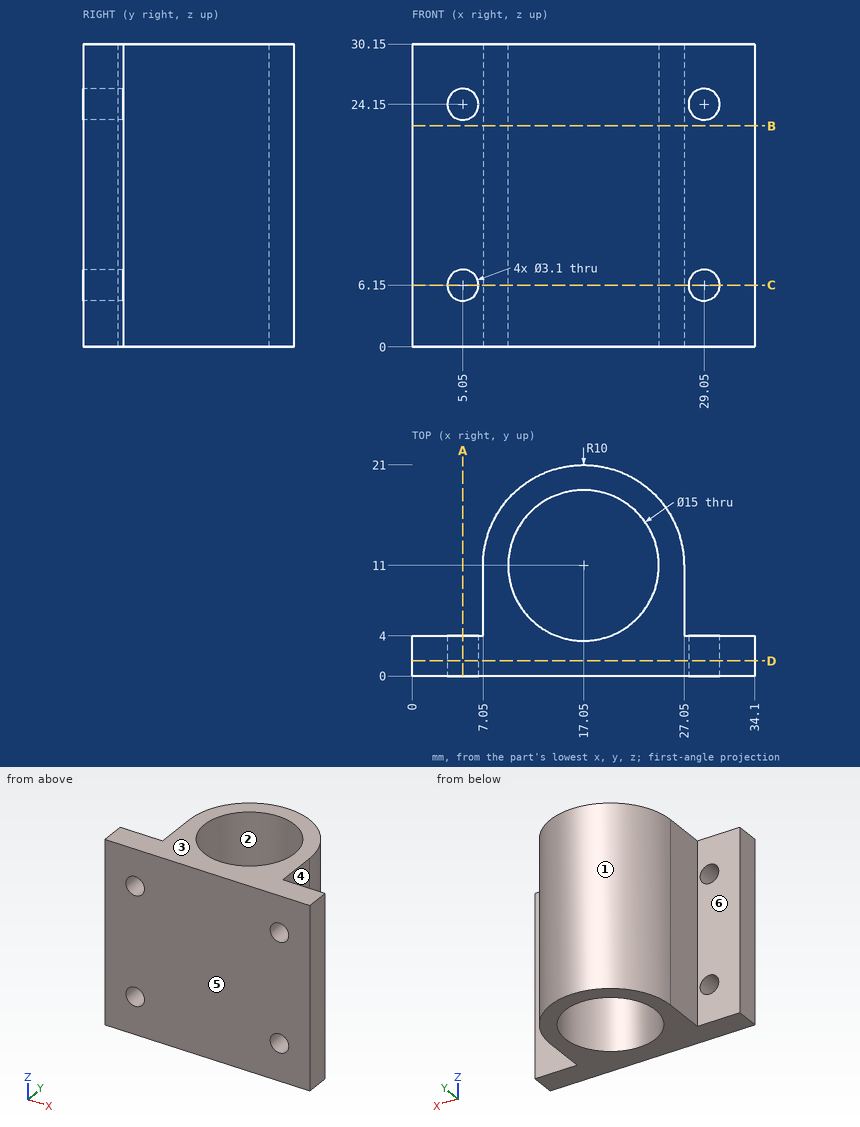
Job drawing, mm, ordinate dimensions from the low corner. One solid piece. A direction names the side the tool comes from. Coordinates: 2 decimals unless noted, no trailing zeros. Write each loop counter-clockwise with the first axis right and the second up, starting at its lowest first coordinate (ties: lowest second). Pieces come first, ordered by that corner, then holes.
Item 1: Slice it at A-A (x = 5.05). Write the cut outline in (y, z), and give its area (3 significant figures).
Item 2: Mould opens along X. For the marked faces 1, 2 and 3 say: released by +X, released by -X, zero draft, split by the parting line, or undercut.
Item 3: Slice it at D-D (y = 1.5). Write the cut outline in (x, z).
Item 4: Slice it at B-B (z = 22). Write the cut outline in (x, y).
Item 5: Probe line 1 (Z direction, x = 5.05, y = 1.75); line 2 (X direction, y = 10.5, z = 13); line 3 (Y direction, x = 21, z = 24). List the from-to ranges inside material, lowest first.
Item 6: Pin check, flat tips, straight feed: pin 1 (3 mm diameter, centred on x = 25.5, z = 5.5, fed in from -Y); pin 2 (8 mm diameter, centred on x = 4.5, z = 9, fed in from +Y); pin 3 (3 mm diameter, centred on x = 29.5, z = 25, fed in from +Y); pin 4 (9 mm diameter, centred on x = 17.05, y = 11, fed in from +Z). Stop position of each tip, or through.
Item 7: Which spindle directions (+Z, -Z, +X, -X, +Y, -Y) get a long thin tool onto all of the face, cutting with end or side? Do the marked faces 4, 5 and 6. Say none if no direction does.
Item 8: Slice it at C-C (z = 6.15). Write the cut outline in (x, y).
Results found:
1. outline: (0, 0) - (4, 0) - (4, 4.6) - (0, 4.6) - close; (0, 7.7) - (4, 7.7) - (4, 22.6) - (0, 22.6) - close; (0, 25.7) - (4, 25.7) - (4, 30.15) - (0, 30.15) - close
1. area: 95.8 mm2
2. face 1: split by the parting line
2. face 2: undercut
2. face 3: zero draft
3. outline: (0, 0) - (34.1, 0) - (34.1, 30.15) - (0, 30.15) - close; hole circle Ø3.1 at (5.05, 6.15); hole circle Ø3.1 at (5.05, 24.15); hole circle Ø3.1 at (29.05, 6.15); hole circle Ø3.1 at (29.05, 24.15)
4. outline: (0, 0) - (34.1, 0) - (34.1, 4) - (27.05, 4) - (27.05, 11) arc R10 ccw to (7.05, 11) - (7.05, 4) - (0, 4) - close; hole circle Ø15 at (17.05, 11)
5. line 1: z = 0 to 4.6, 7.7 to 22.6, 25.7 to 30.15
5. line 2: x = 7.05 to 9.57, 24.53 to 27.05
5. line 3: y = 0 to 4.62, 17.38 to 20.19
6. pin 1: stops at y = 0
6. pin 2: stops at y = 16.19
6. pin 3: stops at y = 4
6. pin 4: passes through
7. face 4: +Z, -Z, +X, +Y
7. face 5: +Z, -Z, +X, -X, -Y
7. face 6: +Z, -Z, -X, +Y
8. outline: (0, 0) - (3.5, 0) - (3.5, 4) - (0, 4) - close; (6.6, 0) - (27.5, 0) - (27.5, 4) - (27.05, 4) - (27.05, 11) arc R10 ccw to (7.05, 11) - (7.05, 4) - (6.6, 4) - close; (30.6, 0) - (34.1, 0) - (34.1, 4) - (30.6, 4) - close; hole circle Ø15 at (17.05, 11)
